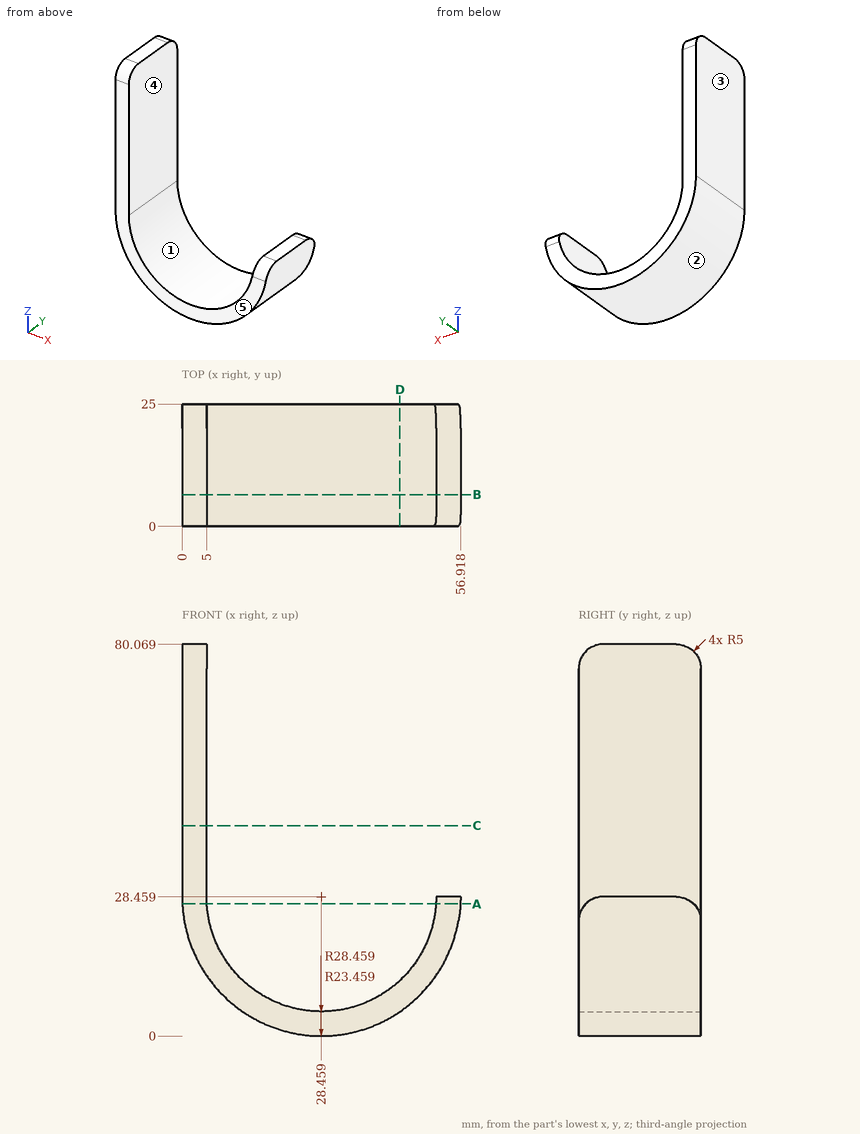
Can you work these out from the drawing? Everything is in mm from the part's minimum corner. A direction names the side the tool comes from. Give positions to 0.01 mm unless a question says otherwise; leave off trailing zeros. Loops run counter-clockwise (first coordinate to the right, second up) from the corner with the lowest first, then second, coordinate; pieces in that order, holes last. Notation, with made-up numbers: M 3.25,62 L 34.25,62 A17 cw 34.25,77 Z; hole C 81,20.25 d3. An arc over 180 degrees is marked long. Put each result on its own line as item: value. Start each with the question number.
(1) I want a section at D-D on x = 44.5. Please give me the cut outline in (y, z), then the cut area to 3 significant figures.
(2) For the marked faces 4 and 5, which set-ups out of +Z, -Z, +X, -X, +Y, -Y let a thin tool reach every point of the face, with its end or its side?
(3) I want a section at A-A on z = 27. Please give me the cut outline in (x, y) (1 decimal), then the cut area to 3 significant figures.
(4) I want a section at B-B on y = 6.5. Please give me the cut outline in (x, z).
(5) I want a section at C-C on z = 43. Please give me the cut outline in (x, y).
(6) I need wall thicknesses on line 1 along X through (y, z) = (9.5, 51.5); line 2 along X through (y, z) = (3.5, 17.5) (1 decimal); line 3 along X through (y, z) = (7.5, 16) (1 decimal). Which ranges of each line are inside material? Lowest first, please. Write a range as [from, to].
(7) If we mould it in two halves opening along X, with no side actions, what happens to the marked faces 1, 2 and 3? For each: +X half, -X half, draft (parallel to the pull), parting line (faces both ways), or undercut.
(8) Will these pins go through, and if not, where does the flat tip stop? pin 1 Ø8 at (x, y) = (50, 18.5) entering from +Z; pin 2 Ø10 at (x, z) = (13.5, 57.5) entering from +Y; pin 3 Ø5 at (x, y) = (16.5, 11) entering from -Z; pin 4 Ø5 at (x, y) = (23.5, 12.5) entering from -Z.
Answer block:
1. outline: M 0,4.95 L 25,4.95 L 25,11.34 L 0,11.34 Z
1. area: 160 mm^2
2. face 4: +Z, +X, +Y, -Y
2. face 5: +Z, -Z, +X, -X, -Y
3. outline: M 0,0 L 5,0 L 5,25 L 0,25 Z; M 51.9,1.5 L 56.9,1.5 L 56.9,23.5 L 51.9,23.5 Z
3. area: 236 mm^2
4. outline: M 0,28.46 A28.46 ccw 56.92,28.46 L 51.92,28.46 A23.46 cw 5,28.46 L 5,80.07 L 0,80.07 Z
5. outline: M 0,0 L 5,0 L 5,25 L 0,25 Z
6. line 1: [0, 5]
6. line 2: [2.2, 7.7], [49.2, 54.7]
6. line 3: [2.9, 8.6], [48.3, 54]
7. face 1: undercut
7. face 2: parting line
7. face 3: -X half
8. pin 1: z = 28.46
8. pin 2: through
8. pin 3: z = 1.62
8. pin 4: z = 0.11
